The model under review builds one solid part; all positions refer to its coordinate system, in mm. A direction names the side the tool comes from. Give positions to 0.01 mm unless a question says otherwise; leave off trailing zeros. Write each loop counter-clockwise with the first axis right and the second up, starting at its lowest first coordinate (ties: lowest second). Pieces come first, ordered by that corner, then holes. Notation, with made-up numbers: (10, -13.75) -> (60, -13.75) arc R34 ccw to (60, 20.25) -> close; hole circle Ø10 at (17.5, -40). An arc over 180 degrees is marked (long way). Use CSV: the item, a comma, the result in double quotes.
```python
from build123d import *

# Parameters (mm, degrees)
BOSS_EXTRUDE1_DEPTH = 2.286
SKETCH3_R           = 1.397
CUT_EXTRUDE1_DEPTH  = 19.288


with BuildPart() as part:
    # Sketch1 → Boss-Extrude1 (new body, symmetric)
    with BuildSketch(Plane.XY):
        Polygon((9.83079784, -10.569522716), (-8.45720216, -10.569522716), (-8.45720216, 6.49008613), (-2.188628559, 6.49008613), (-2.188628559, 0.887867874), (4.211173098, 0.887867874), (4.211173098, 6.49008613), (9.83079784, 6.49008613), align=None)
    extrude(amount=BOSS_EXTRUDE1_DEPTH, both=True)

    # Sketch3 → Cut-Extrude1 (cut, through all)
    with BuildSketch(Plane(origin=(9.83079784, 0, 0), x_dir=(0, 0, -1), z_dir=(1, 0, 0))):
        with Locations((0, 4.20408613)):
            Circle(SKETCH3_R)
    extrude(amount=-CUT_EXTRUDE1_DEPTH, mode=Mode.SUBTRACT)


solid = part.part
```
Q1. Machinability: for faces 4 (the flat face through (1, -10.57, 0)), 5 (the flat face through (-2.189, 2, 0)), which of the approach directions +Z, -Z, +X, -X, +Y, -Y give a long, thin tool a straight path to every point of the face, cutting with its end or side? Answer none if there is none.
Derived:
face 4,"+Z, -Z, +X, -X, -Y"
face 5,"+Z, -Z, +Y"
Q2. Insertion check: pin 1 (2 mm diameter, centred on y = 4.2, z = 0, fed in from -X); pin 2 (2 mm diameter, centred on x = 3, z = 0.5, fed in from +Y). Each pin has a flat end and moves straight along its axis. Give the tip position at first contact, or say it passes through.
Derived:
pin 1,"passes through"
pin 2,"stops at y = 0.89"
Q3. Consider section C-C (x = -2.75). Write out the cut boundary in (y, z).
Derived:
outline,"(-10.57, -2.29) -> (6.49, -2.29) -> (6.49, 2.29) -> (-10.57, 2.29) -> close; hole circle Ø2.79 at (4.2, 0)"
Q4. To check wall thickness, follow probe 1 along Y at (x, z) = (7.1, 0); probe 2 along X at (y, z) = (3.75, 1.45); probe 3 along Y at (x, z) = (-1.25, -0.25). State the ranges of each line that lie inside material, in increasing order.
Derived:
probe 1,"y = -10.57 to 2.81, 5.6 to 6.49"
probe 2,"x = -8.46 to -2.19, 4.21 to 9.83"
probe 3,"y = -10.57 to 0.89"
Q5. The part is to be moulded in two halves that separate along Y. For faces 1 (the flat face through (1, 0.888, 0)), 2 (the flat face through (-8.457, -2, 0)), 3 (the cylindrical face through (-5.279, 3.354, 1.109)), say which applies: pulls with the +Y half, pulls with the -Y half, needs draft (parallel to the pull), parting line crosses it, or undercut.
Derived:
face 1,"pulls with the +Y half"
face 2,"needs draft"
face 3,"undercut"
Q6. Consider section A-A (z = 0). Write out the cut boundary in (x, y), then the cut area to 3 significant figures.
Derived:
outline,"(-8.46, -10.57) -> (9.83, -10.57) -> (9.83, 2.81) -> (4.21, 2.81) -> (4.21, 0.89) -> (-2.19, 0.89) -> (-2.19, 2.81) -> (-8.46, 2.81) -> close; (-8.46, 5.6) -> (-2.19, 5.6) -> (-2.19, 6.49) -> (-8.46, 6.49) -> close; (4.21, 5.6) -> (9.83, 5.6) -> (9.83, 6.49) -> (4.21, 6.49) -> close"
area,"243 mm2"
Q7. Consider section D-D (z = 1.95). Write out the cut boundary in (x, y), then the cut area to 3 significant figures.
Derived:
outline,"(-8.46, -10.57) -> (9.83, -10.57) -> (9.83, 6.49) -> (4.21, 6.49) -> (4.21, 0.89) -> (-2.19, 0.89) -> (-2.19, 6.49) -> (-8.46, 6.49) -> close"
area,"276 mm2"
Q8. Consider section B-B (y = 4.75). Write out the cut boundary in (x, z).
Derived:
outline,"(-8.46, -2.29) -> (-2.19, -2.29) -> (-2.19, -1.29) -> (-8.46, -1.29) -> close; (-8.46, 1.29) -> (-2.19, 1.29) -> (-2.19, 2.29) -> (-8.46, 2.29) -> close; (4.21, -2.29) -> (9.83, -2.29) -> (9.83, -1.29) -> (4.21, -1.29) -> close; (4.21, 1.29) -> (9.83, 1.29) -> (9.83, 2.29) -> (4.21, 2.29) -> close"
